Geometry check sheet. Reference: the model listing, model coordinates, mm. Coordinates: 2 decimals unless noted, no trailing zeros. Write each loop counter-clockwise with the first axis right and the second up, starting at its lowest first coordinate (ties: lowest second). Pieces come first, ordered by that corner, then holes.
from build123d import *

# Parameters (mm, degrees)
SKETCH1_R          = 1.75
SKETCH1_W          = 52
SKETCH1_H          = 5.5
SKETCH1_W_2        = 50
SKETCH1_H_2        = 17.5
SKETCH1_W_3        = 6.5
SKETCH1_H_3        = 6.5
EXTRUDE1_DEPTH     = 4.6
SKETCH2_R          = 1.7
CUT_EXTRUDE1_DEPTH = 163.26527615


with BuildPart() as part:
    # Sketch1 → Extrude1 (new body)
    with BuildSketch(Plane.XY):
        with BuildLine():
            Line((7.924813653, 82.036006536), (136.924813653, 82.036006536))
            ThreePointArc((136.924813653, 82.036006536), (139.046133996, 81.15732688), (139.924813653, 79.036006536))
            Line((139.924813653, 79.036006536), (139.924813653, 8.036006536))
            ThreePointArc((139.924813653, 8.036006536), (139.046133996, 5.914686193), (136.924813653, 5.036006536))
            Line((136.924813653, 5.036006536), (7.924813653, 5.036006536))
            ThreePointArc((7.924813653, 5.036006536), (5.803493309, 5.914686193), (4.924813653, 8.036006536))
            Line((4.924813653, 8.036006536), (4.924813653, 79.036006536))
            ThreePointArc((4.924813653, 79.036006536), (5.803493309, 81.15732688), (7.924813653, 82.036006536))
        make_face()
        with Locations((134.424813653, 76.536006536)):
            Circle(SKETCH1_R, mode=Mode.SUBTRACT)
        with Locations((10.424813653, 76.536006536)):
            Circle(SKETCH1_R, mode=Mode.SUBTRACT)
        with Locations((10.424813653, 15.036006536)):
            Circle(SKETCH1_R, mode=Mode.SUBTRACT)
        with Locations((134.424813653, 15.036006536)):
            Circle(SKETCH1_R, mode=Mode.SUBTRACT)
        with Locations((92.424813653, 74.786006536)):
            Rectangle(SKETCH1_W, SKETCH1_H, mode=Mode.SUBTRACT)
        with Locations((81.924813653, 36.786006536)):
            Rectangle(SKETCH1_W_2, SKETCH1_H_2, mode=Mode.SUBTRACT)
        with Locations((100.174813653, 54.286006536)):
            Rectangle(SKETCH1_W_3, SKETCH1_H_3, mode=Mode.SUBTRACT)
    extrude(amount=EXTRUDE1_DEPTH)

    # Sketch2 → Cut-Extrude1 (cut, through all)
    with BuildSketch(Plane(origin=(0, 0, 0), x_dir=(-1, 0, 0), z_dir=(0, 0, -1))):
        with Locations((-50.924813653, 25.036006536)):
            Circle(SKETCH2_R)
        with Locations((-9.924813653, 25.036006536)):
            Circle(SKETCH2_R)
    extrude(amount=-CUT_EXTRUDE1_DEPTH, mode=Mode.SUBTRACT)


solid = part.part
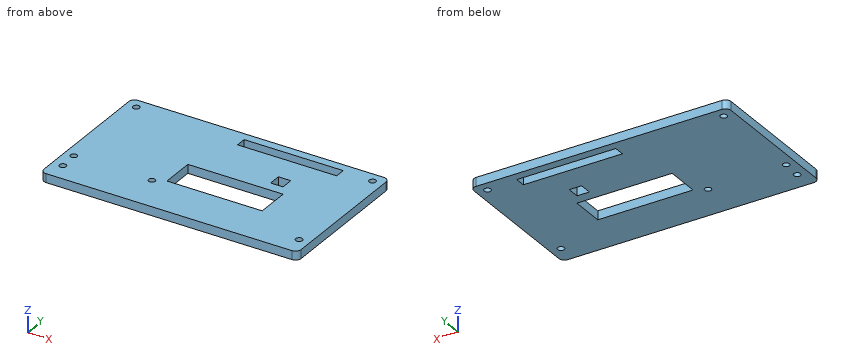
1. Sectioned sample at D-D, the plane z = 3.7. Give the number of separate pieces and of enclosed holes in the cut face, and give its area (3 significant figures).
Computed values:
separate pieces: 1
enclosed holes: 9
area: 9,130 mm2
2. Sectioned sample at C-C, the plane x = 80. Record the boundary of the cut face in (y, z), and give its area (3 significant figures).
Computed values:
outline: (5.04, 0) - (28.04, 0) - (28.04, 4.6) - (5.04, 4.6) - close; (45.54, 0) - (72.04, 0) - (72.04, 4.6) - (45.54, 4.6) - close; (77.54, 0) - (82.04, 0) - (82.04, 4.6) - (77.54, 4.6) - close
area: 248 mm2
3. Thickness scan on line 1 along Y through (x, z) = (95.5, 3.95); line 2 along X through (y, z) = (38, 2.45); line 3 along X through (y, z) = (14, 4.45). Record the ranges inside material, lowest first.
Computed values:
line 1: y = 5.04 to 28.04, 45.54 to 72.04, 77.54 to 82.04
line 2: x = 4.92 to 56.92, 106.92 to 139.92
line 3: x = 4.92 to 9.01, 11.84 to 133.01, 135.84 to 139.92
4. Sectioned sample at B-B, the plane x = 64. Record the boundary of the cut face in (y, z).
Computed values:
outline: (5.04, 0) - (28.04, 0) - (28.04, 4.6) - (5.04, 4.6) - close; (45.54, 0) - (82.04, 0) - (82.04, 4.6) - (45.54, 4.6) - close
5. Sectioned sample at A-A, the plane y = 36.5. Record the boundary of the cut face in (x, z).
Computed values:
outline: (4.92, 0) - (56.92, 0) - (56.92, 4.6) - (4.92, 4.6) - close; (106.92, 0) - (139.92, 0) - (139.92, 4.6) - (106.92, 4.6) - close
